Build history of the part. All positions in model axes, mm. Face numbers are marked on the shaded views. A direction names the side the tool comes from. Round coordinates to 2 decimals unless told otherwise and drop trailing zeros. Write each loop counter-clockwise with the first axis right and the second up, starting at its lowest first coordinate (ties: lowest second). Pieces come first, ordered by that corner, then holes. Notation, with made-up numbers: (-16.5, 6) - (15.5, 6) arc R22 cw to (15.5, 18) - close; hole circle Ø1 at (86.5, 1). An arc over 180 degrees is marked (long way). Write each question's results on one line, items separated by ' | '.
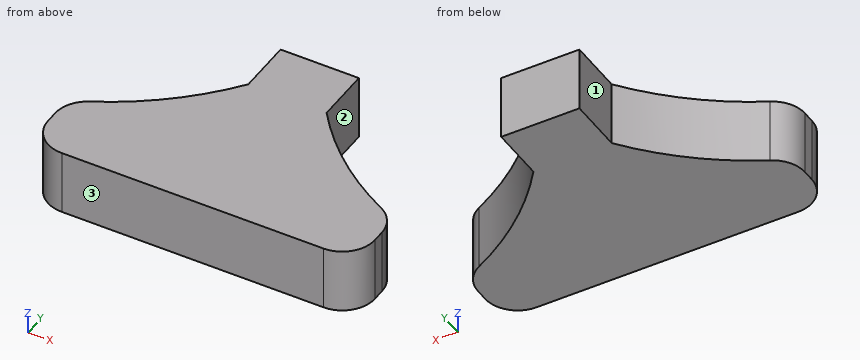
Solid Edge part; units mm, degrees
sketch "Sketch1" plane through (0, 0, 0) normal (0, 0, 1) x (1, 0, 0)
  line L0 (-50.11, -33.5) -> (50.11, -33.5)
  line L1 (50.11, -33.5) -> (50.11, 33.5)
  line L2 (50.11, 33.5) -> (-50.11, 33.5)
  line L3 (-50.11, 33.5) -> (-50.11, -33.5)
extrude "Protrusion1" add sketch "Sketch1" against normal blind 20
sketch "Sketch2" plane through (0, 0, 0) normal (0, 0, 1) x (1, 0, 0)
  line L0 (-50.11, 33.5) -> (-12, 33.5)
  line L1 (-12, 33.5) -> (-12, 16.5)
  line L2 (-12, 16.5) -> (-50.11, 16.5)
  line L3 (-50.11, 16.5) -> (-50.11, 33.5)
extrude "ExtrudedCutout_1" cut sketch "Sketch2" against normal blind 20
sketch "Sketch3" plane through (0, 0, 0) normal (0, 0, 1) x (1, 0, 0)
  line L0 (50.11, 33.5) -> (12, 33.5)
  line L1 (12, 33.5) -> (12, 16.5)
  line L2 (12, 16.5) -> (50.11, 16.5)
  line L3 (50.11, 16.5) -> (50.11, 33.5)
extrude "ExtrudedCutout_2" cut sketch "Sketch3" against normal blind 20
sketch "Sketch4" plane through (0, 0, 0) normal (0, 0, 1) x (1, 0, 0)
  arc A0 (-50.11, -13.5) -> (-12, 16.5) centre (-87.2296, 72.8605) ccw
  line L0 (-12, 16.5) -> (-50.11, 16.5)
  line L1 (-50.11, 16.5) -> (-50.11, -13.5)
extrude "ExtrudedCutout_3" cut sketch "Sketch4" against normal blind 20
sketch "Sketch5" plane through (0, 0, 0) normal (0, 0, 1) x (1, 0, 0)
  arc A0 (50.11, -13.5) -> (12, 16.5) centre (87.2296, 72.8605) cw
  line L0 (12, 16.5) -> (50.11, 16.5)
  line L1 (50.11, 16.5) -> (50.11, -13.5)
extrude "ExtrudedCutout_4" cut sketch "Sketch5" against normal blind 20
fillet "Round_1" radius 10 4 edges at (50.11, -13.5, -10) (50.11, -33.5, -10) (-50.11, -33.5, -10) (-50.11, -13.5, -10)
(1) Slice it at C-C, the plane x = 17.5. Write the cut outline in (y, z).
Worked answers:
outline: (-33.5, -20) - (9.82, -20) - (9.82, 0) - (-33.5, 0) - close
(2) Flat gauge pins, fed straight in: pin 1 Ø8.5 at (y, z) = (28.5, -5.5) entering from +X; pin 2 Ø12 at (x, z) = (37, -16.5) entering from +Y; pin 3 Ø10 at (y, z) = (-16.5, -3) entering from -X. Where does each tip first touch, or does it go through?
Worked answers:
pin 1: stops at x = 12 | pin 2: stops at y = -2.47 | pin 3: stops at x = -50.11
(3) Slice it at B-B, the plane y = 23. Write the cut outline in (x, z).
Worked answers:
outline: (-12, -20) - (12, -20) - (12, 0) - (-12, 0) - close
(4) Slice it at A-A, the plane z = -1.75. Write the cut outline in (x, y), and give its area (3 significant figures).
Worked answers:
outline: (-50.11, -23.5) arc R10 ccw to (-40.11, -33.5) - (40.11, -33.5) arc R10 ccw to (50.11, -23.5) - (50.11, -19.85) arc R10 ccw to (44.64, -10.94) arc R94 cw to (12, 16.5) - (12, 33.5) - (-12, 33.5) - (-12, 16.5) arc R94 cw to (-44.64, -10.94) arc R10 ccw to (-50.11, -19.85) - close | area: 4,010 mm2
(5) Tool access for the marked faces 1, 2 and 3: list every direction of +Z, -Z, +X, -X, +Y, -Y with a clear straight run to the whole face (end or side of a thin tool).
Worked answers:
face 1: +Z, -Z, -X, +Y | face 2: +Z, -Z, +X, +Y | face 3: +Z, -Z, +X, -X, -Y
(6) Drill centre lines: probe 1 along X at (y, z) = (27, -12.75); probe 2 along Y at (x, z) = (-27, -4.5); probe 3 along X at (y, z) = (2, -12.5). Where is each one in solid material? Low to high. Write a range as [from, to].
Worked answers:
probe 1: x = [-12, 12] | probe 2: y = [-33.5, 0.69] | probe 3: x = [-25.47, 25.47]
